For this review, take the finished solid that the model builds, in its own axes (mm). Round coordinates to 2 decimals unless told otherwise and drop trailing zeros. Order: outer loops, then holes, each group sorted by start corner. A loop starts at its lowest first (then second) coordinate and runs counter-clockwise, first axis right, second up. Notation, with made-up numbers: M -40,-5 L -21,-5 A30 cw -21,20 Z; hole C -34,-11.5 d3. An arc over 180 degrees is marked long. Put each result on its own line as item: value.
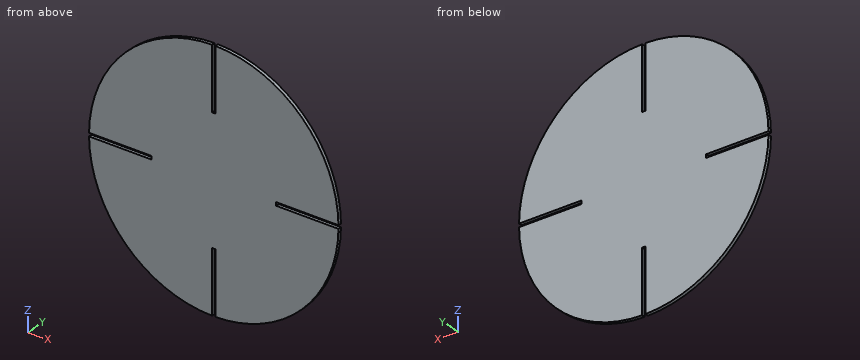
from build123d import *

# Parameters (mm, degrees)
F1_DEPTH = 2


with BuildPart() as f1:
    # F0 (on Front) → F1 (new body)
    with BuildSketch(Plane.XZ):
        with BuildLine():
            Line((-1, 37.5), (-1, 74.993333))
            ThreePointArc((-1, 74.993333), (-53.033009, 53.033009), (-74.993333, 1))
            Line((-74.993333, 1), (-37.5, 1))
            Line((-37.5, 1), (-37.5, 0))
            Line((-37.5, 0), (-37.5, -1))
            Line((-37.5, -1), (-74.993333, -1))
            ThreePointArc((-74.993333, -1), (-53.033009, -53.033009), (-1, -74.993333))
            Line((-1, -74.993333), (-1, -37.5))
            Line((-1, -37.5), (1, -37.5))
            Line((1, -37.5), (1, -74.993333))
            ThreePointArc((1, -74.993333), (53.033009, -53.033009), (74.993333, -1))
            Line((74.993333, -1), (37.5, -1))
            Line((37.5, -1), (37.5, 0))
            Line((37.5, 0), (37.5, 1))
            Line((37.5, 1), (74.993333, 1))
            ThreePointArc((74.993333, 1), (53.033009, 53.033009), (1, 74.993333))
            Line((1, 74.993333), (1, 37.5))
            Line((1, 37.5), (-1, 37.5))
        make_face()
    extrude(amount=F1_DEPTH)


solid = f1.part
(1) Insertion check: pin 1 Ø1 at (x, y) = (0, -0.5) entering from +Z; pin 2 Ø1 at (x, y) = (-65.5, -1.5) entering from +Z; pin 3 Ø1 at (y, z) = (-1, 57.5) entering from +X. Each pin has a flat end and moves straight along its axis. Give the tip position at first contact, or say it passes through.
A:
pin 1: stops at z = 37.5
pin 2: stops at z = 37.42
pin 3: stops at x = 48.74
(2) Add section D-D on z = -21. Give the boundary of the cut face in (x, y), then the cut area to 3 significant figures.
A:
outline: M -72,-2 L 72,-2 L 72,0 L -72,0 Z
area: 288 mm2
(3) Add section A-A on z = -42. Give the boundary of the cut face in (x, y).
A:
outline: M -62.14,-2 L -1,-2 L -1,0 L -62.14,0 Z; M 1,-2 L 62.14,-2 L 62.14,0 L 1,0 Z
(4) To check wall thickness, follow L1, parallel to X at y = -1.5, z = 2.5; L2, parallel to Z at x = -44.5, y = -1.75; L3, parallel to X at y = -0.5, z = 45.5. State the ranges of each line that lie inside material, in increasing order.
A:
L1: x = -74.96 to 74.96
L2: z = -60.37 to -1, 1 to 60.37
L3: x = -59.62 to -1, 1 to 59.62
(5) Add section B-B on y = -0.55. Give the boundary of the cut face in (x, z), then the cut area to 3 significant figures.
A:
outline: M -74.99,-1 A75 ccw -1,-74.99 L -1,-37.5 L 1,-37.5 L 1,-74.99 A75 ccw 74.99,-1 L 37.5,-1 L 37.5,1 L 74.99,1 A75 ccw 1,74.99 L 1,37.5 L -1,37.5 L -1,74.99 A75 ccw -74.99,1 L -37.5,1 L -37.5,-1 Z
area: 17,400 mm2
(6) Add section C-C on x = -49. Give the boundary of the cut face in (y, z).
A:
outline: M -2,-56.78 L 0,-56.78 L 0,-1 L -2,-1 Z; M -2,1 L 0,1 L 0,56.78 L -2,56.78 Z
